Autodesk Inventor part; units mm, degrees
ref_plane "YZ Plane" through (0, 0, 0) normal (1, 0, 0) x (0, 1, 0)
ref_plane "XZ Plane" through (0, 0, 0) normal (0, 1, 0) x (-1, 0, 0)
ref_plane "XY Plane" through (0, 0, 0) normal (0, 0, 1) x (1, 0, 0)
sketch "Sketch1" plane through (0, 0, 0) normal (1, 0, 0) x (0, 1, 0)
  line L0 (14.9656, 6.7345) -> (-10.4344, 6.7345)
  line L1 (-10.4344, 6.7345) -> (-10.4344, -5.9655)
  line L2 (-10.4344, -5.9655) -> (14.9656, -5.9655)
  line L3 (14.9656, -5.9655) -> (14.9656, 6.7345)
  point P0 (0, 0)
  dimension "d0" = 25.4
  dimension "d1" = 12.7
extrude "Extrusion1" add sketch "Sketch1" along normal blind 6.35
sketch "Sketch2" plane through (6.35, 0, 0) normal (1, 0, 0) x (0, 0, -1)
  circle A0 centre (-4.1568, 12.913) radius 1.5875
  line L0 (-6.7345, 14.9656) -> (-6.7345, -10.4344)
  line L1 (5.9655, 14.9656) -> (-6.7345, 14.9656)
  circle A1 centre (2.1932, 12.913) radius 1.5875
  circle A2 centre (-4.1568, -6.137) radius 1.5875
  circle A3 centre (2.1932, -6.137) radius 1.5875
  point P0 (0, 0)
  dimension "d4" = 3.175
  dimension "d9" = 6.35
  dimension "d12" = 19.05
extrude "Extrusion2" cut sketch "Sketch2" against normal blind 6.35
equation "\"d1\" = 0.5 * d0"
equation "\"d2\" = 0.5 * d1"
equation "\"d4\" = 0.5 * d2"
equation "\"d15\" = 0.5 * d1"
properties part number "8.2a"
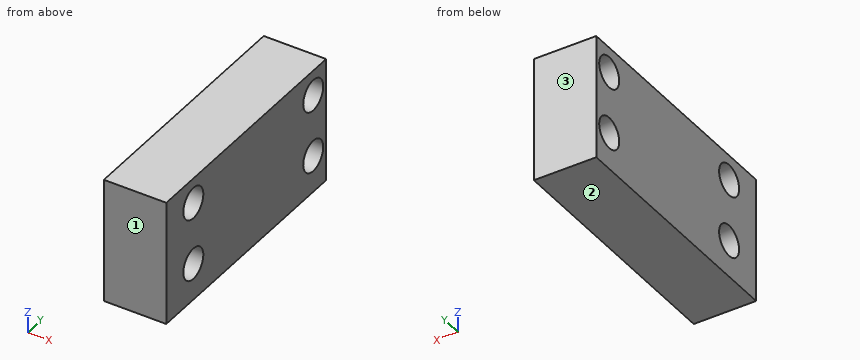
Part model, mm, in its own coordinate system. Face numbers are marked on the shaded views. Give positions to 0.01 mm unless a question says otherwise; leave off trailing zeros. Loops run counter-clockwise (first coordinate to the right, second up) from the corner with the lowest first, then second, coordinate; pieces in that order, holes last. Notation, with made-up numbers: M 63,11.25 L 80,11.25 A33 cw 80,47.25 Z; hole C -31.5,25 d7. An arc over 180 degrees is marked long. Return JSON: item names as keys, results as strings.
1) Saw through at A-A, the plane z = -3. List the corners of the cut face in (x, y).
Calculated:
{"outline": "M 0,-10.43 L 6.35,-10.43 L 6.35,-7.5 L 0,-7.5 Z; M 0,-4.77 L 6.35,-4.77 L 6.35,11.55 L 0,11.55 Z; M 0,14.28 L 6.35,14.28 L 6.35,14.97 L 0,14.97 Z"}
2) Pull direction Y, two halves, no side cores. Call the marked faces 1, 2 and 3: released by +Y, released by -Y, zero draft, split by the parting line, or undercut.
Calculated:
{"face 1": "released by -Y", "face 2": "zero draft", "face 3": "released by +Y"}
3) Drill centre lines: line 1 (Z direction, x = 1.5, y = 13); line 2 (Y direction, x = 0.75, z = 5.5); line 3 (Y direction, x = 2.25, z = -1). Where is each one in solid material? Low to high.
Calculated:
{"line 1": "z = -5.97 to -3.78, -0.61 to 2.57, 5.74 to 6.73", "line 2": "y = -10.43 to -6.98, -5.29 to 12.07, 13.76 to 14.97", "line 3": "y = -10.43 to -7.18, -5.09 to 11.87, 13.96 to 14.97"}
4) Saw through at B-B, the plane y = -6.5. List the corners of the cut face in (x, z), then the cut area to 3 significant figures.
Calculated:
{"outline": "M 0,-5.97 L 6.35,-5.97 L 6.35,-3.74 L 0,-3.74 Z; M 0,-0.65 L 6.35,-0.65 L 6.35,2.61 L 0,2.61 Z; M 0,5.7 L 6.35,5.7 L 6.35,6.73 L 0,6.73 Z", "area": "41.4 mm2"}
5) Saw through at C-C, the plane x = 5.75. List the corners of the cut face in (y, z) (1 decimal), then the cut area to 3 significant figures.
Calculated:
{"outline": "M -10.4,-6 L 15,-6 L 15,6.7 L -10.4,6.7 Z; hole C -6.1,-2.2 d3.2; hole C -6.1,4.2 d3.2; hole C 12.9,-2.2 d3.2; hole C 12.9,4.2 d3.2", "area": "291 mm2"}
